Verification items for this drawing (mm, ordinates from the low corner). A direction names the side the tool comes from. Round coordinates to 2 decimals unless told otherwise and drop trailing zeros. Order: outer loops, then holes, each group sorted by start corner. A loop starts at its lowest first (then second) coordinate and runs counter-clockwise, first axis right, second up. Notation, with made-up numbers: (86, 1) -> (117, 1) arc R14 cw to (117, 17) -> close; hole circle Ø10 at (21, -28). An arc over 180 degrees is marked (long way). Put each result on its own line as item: value.
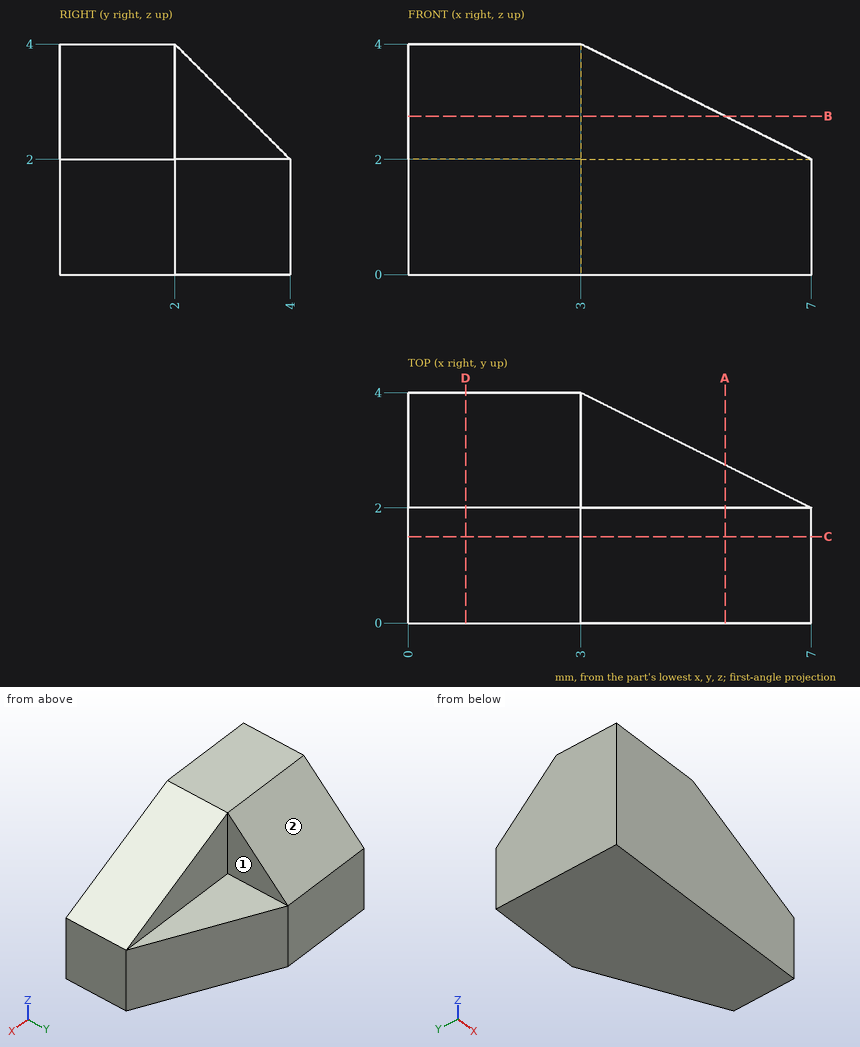
Item 1: Material ranges on L1, parallel to Y at x = 4.25, z = 2.6; L2, parallel to X at y = 3.35, z = 2.15, recorded low to high. Write a range as [from, to].
Check sheet entries:
L1: y = [0, 2]
L2: x = [0, 3]
Item 2: Gauge pin test, flat ends, axial feed: pin 1 Ø1.6 at (x, y) = (5.5, 3) entering from +Z; pin 2 Ø2 at (x, z) = (5.5, 2.5) entering from +Y; pin 3 Ø0.6 at (y, z) = (3, 3) entering from +X. Record the tip position at first contact, or that the pin passes through.
Check sheet entries:
pin 1: stops at z = 2
pin 2: stops at y = 3.18
pin 3: stops at x = 3
Item 3: Tool access check on the marked faces 1 and 2. Record the directions out of +Z, -Z, +X, -X, +Y, -Y that give a thin tool (end or side, any length) a straight path to the whole face; none if there is none.
Check sheet entries:
face 1: +Z, +X, +Y
face 2: +Z, +X, -X, +Y
Item 4: Section check D-D on x = 1. Record the boundary of the cut face in (y, z), then the cut area to 3 significant figures.
Check sheet entries:
outline: (0, 0) -> (4, 0) -> (4, 2) -> (2, 4) -> (0, 4) -> close
area: 14.0 mm^2
Item 5: Section check B-B on z = 2.75. Record the boundary of the cut face in (x, y), then the cut area to 4 significant figures.
Check sheet entries:
outline: (0, 0) -> (5.5, 0) -> (5.5, 2) -> (3, 2) -> (3, 3.25) -> (0, 3.25) -> close
area: 14.75 mm^2
Item 6: Section check C-C on y = 1.5. Record the boundary of the cut face in (x, z), then the cut area to 3 significant figures.
Check sheet entries:
outline: (0, 0) -> (7, 0) -> (7, 2) -> (3, 4) -> (0, 4) -> close
area: 24.0 mm^2
Item 7: Section check A-A on x = 5.5. Record the boundary of the cut face in (y, z).
Check sheet entries:
outline: (0, 0) -> (2.75, 0) -> (2.75, 2) -> (2, 2) -> (2, 2.75) -> (0, 2.75) -> close
